from build123d import *

# Parameters (mm, degrees)
BOSS_EXTRUDE1_DEPTH      = 4
CUT_EXTRUDE1_REACH       = 6
SKETCH3_W                = 6
SKETCH3_H                = 10
SKETCH4_W                = 2
SKETCH4_H                = 1.5
BOSS_EXTRUDE2_DEPTH      = 4.75
BOSS_EXTRUDE2_DEPTH_BACK = 4.75
SKETCH5_W                = 3
SKETCH5_H                = 6
CUT_EXTRUDE2_DEPTH       = 0.8
SKETCH6_W                = 2
SKETCH6_H                = 1.1
CUT_EXTRUDE3_DEPTH       = 67.5
CHAMFER3_SIZE            = 0.4
CHAMFER3_SIZE2           = 1.098990968
CHAMFER4_SIZE            = 0.7
CHAMFER4_SIZE2           = 1.923234194
CHAMFER4_PART_2_SIZE     = 0.7
CHAMFER4_PART_2_SIZE2    = 1.923234194


with BuildPart() as part:
    # Sketch1 → Boss-Extrude1 (new body)
    with BuildSketch(Plane(origin=(0, 0, 0), x_dir=(1, 0, 0), z_dir=(0, 1, 0))):
        Polygon((-51.75, 24.75), (-51.75, 41.75), (51.75, 41.75), (51.75, -41.75), (-51.75, -41.75), (-51.75, -24.75), (-53.75, -24.75), (-53.75, -15.25), (-51.75, -15.25), (-51.75, 15.25), (-53.75, 15.25), (-53.75, 24.75), align=None)
    extrude(amount=BOSS_EXTRUDE1_DEPTH)

    # Sketch3 → Cut-Extrude1 (cut, up to next)
    with BuildSketch(Plane(origin=(0, 4, 0), x_dir=(1, 0, 0), z_dir=(0, 1, 0)), mode=Mode.PRIVATE) as cut_extrude1_sk1:
        with Locations((48.75, 0)):
            Rectangle(SKETCH3_W, SKETCH3_H)
    cut_extrude1_tool1 = extrude(cut_extrude1_sk1.sketch, amount=-CUT_EXTRUDE1_REACH, mode=Mode.PRIVATE) & part.part
    add(cut_extrude1_tool1.solids().sort_by_distance((48.75, 4, 0))[0], mode=Mode.SUBTRACT)

    # Sketch4 → Boss-Extrude2 (add, two sides)
    with BuildSketch(Plane.XY) as boss_extrude2_sk:
        with BuildLine():
            Line((44.75, 4), (45.75, 4))
            Line((45.75, 4), (45.75, 9.863040099))
            ThreePointArc((45.75, 9.863040099), (46.689528886, 10.982727024), (47.955352731, 10.251903287))
            Line((47.955352731, 10.251903287), (50.321851993, 3.75))
            Line((50.321851993, 3.75), (48.25, 3.75))
            Line((48.25, 3.75), (48.25, 1.25))
            Line((48.25, 1.25), (51.75, 1.25))
            Line((51.75, 1.25), (51.75, 2.75))
            Line((51.75, 2.75), (48.895045351, 10.59392343))
            ThreePointArc((48.895045351, 10.59392343), (46.515880709, 11.967534777), (44.75, 9.863040099))
            Line((44.75, 9.863040099), (44.75, 4))
        make_face()
        with Locations((52.75, 2)):
            Rectangle(SKETCH4_W, SKETCH4_H)
    extrude(amount=BOSS_EXTRUDE2_DEPTH)
    extrude(boss_extrude2_sk.sketch, amount=-BOSS_EXTRUDE2_DEPTH_BACK)

    # Sketch5 → Cut-Extrude2 (cut)
    with BuildSketch(Plane.XZ.offset(-1.25)):
        with Locations((50.25, 0)):
            Rectangle(SKETCH5_W, SKETCH5_H)
    extrude(amount=-CUT_EXTRUDE2_DEPTH, mode=Mode.SUBTRACT)

    # Sketch6 → Cut-Extrude3 (cut, through all)
    with BuildSketch(Plane.XY.offset(24.75)):
        with Locations((-52.75, 3.45)):
            Rectangle(SKETCH6_W, SKETCH6_H)
        with Locations((-52.75, 0.55)):
            Rectangle(SKETCH6_W, SKETCH6_H)
    extrude(amount=-CUT_EXTRUDE3_DEPTH, mode=Mode.SUBTRACT)

    # Chamfer3
    chamfer3_edges = [part.edges().sort_by_distance(p)[0] for p in [
        (53.75, 2.75, 0),
        (53.75, 2, 4.75),
        (53.75, 1.25, 0),
        (53.75, 2, -4.75),
    ]]
    chamfer3_side = [part.faces().sort_by_distance(p)[0] for p in [
        (53.75, 2, 0),
    ]]
    chamfer(chamfer3_edges, length=CHAMFER3_SIZE, length2=CHAMFER3_SIZE2, reference=chamfer3_side[0])

    # Chamfer4
    chamfer4_edges = [part.edges().sort_by_distance(p)[0] for p in [
        (-53.75, 2, 15.25),
        (-53.75, 2.9, 20),
        (-53.75, 1.1, 20),
        (-53.75, 2, 24.75),
    ]]
    chamfer4_side = [part.faces().sort_by_distance(p)[0] for p in [
        (-53.75, 2, 20),
    ]]
    chamfer(chamfer4_edges, length=CHAMFER4_SIZE, length2=CHAMFER4_SIZE2, reference=chamfer4_side[0])

    # Chamfer4 part 2
    chamfer4_part_2_edges = [part.edges().sort_by_distance(p)[0] for p in [
        (-53.75, 2, -15.25),
        (-53.75, 2, -24.75),
        (-53.75, 2.9, -20),
        (-53.75, 1.1, -20),
    ]]
    chamfer4_part_2_side = [part.faces().sort_by_distance(p)[0] for p in [
        (-53.75, 2, -20),
    ]]
    chamfer(chamfer4_part_2_edges, length=CHAMFER4_PART_2_SIZE, length2=CHAMFER4_PART_2_SIZE2, reference=chamfer4_part_2_side[0])


solid = part.part
Geometry: final body of the model. Coordinates: model frame, mm. A direction names the side the tool comes from. Give positions to 0.01 mm unless a question says otherwise; leave off trailing zeros. Write each loop counter-clockwise with the first axis right and the second up, starting at its lowest first coordinate (ties: lowest second). Pieces come first, ordered by that corner, then holes.
(1) Cut plane B-B, the plane z = 18.5. Return loops of the section in (x, y), then the cut area to 3 significant figures.
(2) First-contact query: P1, Ø3.5, axis at x = 49.5, z = -1, coming from the -Y side; P2, Ø1.3, axis at x = 50.5, z = 2, coming from the -Y side; P3, Ø4, axis at y = 8.5, z = -5, coming from the -X side; P4, Ø3, axis at x = 42.5, y = 10.5, coming from the +Z side. Flat tips, straight axial feed; report the tip coordinate or a pass-through.
(3) Cut plane A-A, the plane y = 8.5. Return loops of the section in (x, z).
(4) Cut plane C-C, the plane x = -23. Return loops of the section in (y, z).
(5) Mould query, pull axis Y, two halves, no side actions, for faces 1 (the flat face through (49, 2, 5)), 2 (the flat face through (1, 0, -1)), 3 (the flat face through (49.12, 7.05, 0.07)). Classes: released by +Y, released by -Y, zero draft, split by the parting line, or undercut.
(6) Access query for faces 4 (the flat face through (49, 3.75, 0)), 5 (the flat face through (50, 2.05, 0)), 6 (the flat face through (49, 2, -5)), 7 (the flat face through (44.75, 7, 0)). Directions: +Z, -Z, +X, -X, +Y, -Y. A direction counts if a zero-diameter tool reaches every point of the face in a straight line with its end or side. Return the directions, or none.
(7) Ray query, line 1 (Y direction, x = 24.5, z = -25.5); line 2 (X direction, y = 1, z = -37.5); line 3 (X direction, y = 11.25, z = -4). Return the intervals inside material, ascending.
(8) Cut plane D-D, the plane z = 0. Return loops of the section in (x, y).
Values follow:
1. outline: (-53.75, 1.8) - (-51.83, 1.1) - (-51.75, 1.1) - (-51.75, 0) - (51.75, 0) - (51.75, 4) - (-51.75, 4) - (-51.75, 2.9) - (-51.83, 2.9) - (-53.75, 2.2) - close
1. area: 416 mm2
2. P1: stops at y = 1.25
2. P2: stops at y = 2.05
2. P3: stops at x = 44.75
2. P4: passes through
3. outline: (44.75, -4.75) - (45.75, -4.75) - (45.75, 4.75) - (44.75, 4.75) - close; (48.59, -4.75) - (49.66, -4.75) - (49.66, 4.75) - (48.59, 4.75) - close
4. outline: (0, -41.75) - (4, -41.75) - (4, 41.75) - (0, 41.75) - close
5. face 1: zero draft
5. face 2: released by -Y
5. face 3: undercut
6. face 4: none
6. face 5: -Y
6. face 6: +X, +Y, -Y
6. face 7: +Z, -Z, -X, +Y
7. line 1: y = 0 to 4
7. line 2: x = -51.75 to 51.75
7. line 3: x = 45.26 to 48.51
8. outline: (-51.75, 0) - (45.75, 0) - (45.75, 9.86) arc R1.14 cw to (47.96, 10.25) - (50.32, 3.75) - (48.25, 3.75) - (48.25, 1.25) - (48.75, 1.25) - (48.75, 2.05) - (51.75, 2.05) - (51.75, 1.25) - (52.65, 1.25) - (53.75, 1.65) - (53.75, 2.35) - (52.65, 2.75) - (51.75, 2.75) - (48.9, 10.59) arc R2.14 ccw to (44.75, 9.86) - (44.75, 4) - (-51.75, 4) - close
